Design review of the part built by this model. Coordinates are the model's own, in mm. A direction names the side the tool comes from. Round coordinates to 2 decimals unless told otherwise and drop trailing zeros. Loops run counter-clockwise (first coordinate to the right, second up) from the corner with the lowest first, then second, coordinate; pieces in that order, holes last. Notation, with made-up numbers: (0.25, 46) - (18.25, 46) arc R16 ccw to (18.25, 50) - close; hole circle Ø1 at (11.5, 62). An arc over 180 degrees is marked (long way). Use one line per item in the form item = value. Start each with the question number.
(1) For pin 1 (5 mm diameter, centred on y = -7, z = -5, fed in from -X); pin 2 (4 mm diameter, centred on x = 3, y = -5.5, fed in from -Z), all flat-tipped, find the tip position at first contact; note any pin that passes through.
(2) Wall thickness on probe 1 along Y at (x, z) = (5, 5); probe 2 along Z at (x, y) = (18.15, -5); probe 3 along Z at (x, y) = (17.75, -5.75): over which ranges is each line inside the solid? List them lowest first. Write a range as [from, to].
(3) We need section D-D, the plane z = -7.25. Write out the cut boundary in (x, y), then the cut area to 3 significant figures.
(4) The part is to be moulded in two halves that separate along Y. For faces 1 (the cylindrical face through (18.52, -5.27, -8.47)), 2 (the cylindrical face through (7.385, -4.249, 4.93)), 3 (the flat face through (10, 0, 5)), 4 (the flat face through (20, -5, 0)), say which applies: released by +Y, released by -Y, zero draft, split by the parting line, or undercut.
(5) We need section C-C, the plane x = 5. Write out the cut boundary in (y, z).
(6) Machinability: for faces 5 (the flat face through (8, -5, 0)), 6 (the flat face through (0, -5, 5)), which of the approach directions +Z, -Z, +X, -X, +Y, -Y give a long, thin tool a straight path to every point of the face, cutting with its end or side? Answer none if there is none.
(7) We need section A-A, the plane y = -5. Write out the cut boundary in (x, z), then the cut area to 4 significant figures.
(8) We need section B-B, the plane z = 7. Write out the cut boundary in (x, y), then the cut area to 3 significant figures.
from build123d import *

# Parameters (mm, degrees)
F0_W     = 20
F0_H     = 10
F0_R     = 2.5
F1_DEPTH = 10
F2_W     = 3
F2_H     = 10
F3_DEPTH = 10
F4_R     = 1.25
F5_DEPTH = 3


with BuildPart() as f1:
    # F0 (on Top) → F1 (new body)
    with BuildSketch(Plane.XY):
        with Locations((10, -5)):
            Rectangle(F0_W, F0_H)
        with Locations((5, -5)):
            Circle(F0_R, mode=Mode.SUBTRACT)
    extrude(amount=F1_DEPTH)

    # F2 (on face) → F3 (join)
    with BuildSketch(Plane(origin=(0, 0, 0), x_dir=(1, 0, 0), z_dir=(0, 0, -1))):
        with Locations((18.5, 5)):
            Rectangle(F2_W, F2_H)
    extrude(amount=F3_DEPTH)

    # F4 (on face) → F5 (cut, through all)
    with BuildSketch(Plane.YZ.offset(20)):
        with Locations((-5, -7.25)):
            Circle(F4_R)
    extrude(amount=-F5_DEPTH, mode=Mode.SUBTRACT)


solid = f1.part
Data:
q1.pin_1 = 17
q1.pin_2 = 0
q2.probe_1 = [-10, -7.5], [-2.5, 0]
q2.probe_2 = [-10, -8.5], [-6, 10]
q2.probe_3 = [-10, -8.25], [-6.25, 10]
q3.outline = (17, -10) - (20, -10) - (20, -6.25) - (17, -6.25) - close; (17, -3.75) - (20, -3.75) - (20, 0) - (17, 0) - close
q3.area = 22.5 mm^2
q4.face_1 = undercut
q4.face_2 = undercut
q4.face_3 = released by +Y
q4.face_4 = zero draft
q5.outline = (-10, 0) - (-7.5, 0) - (-7.5, 10) - (-10, 10) - close; (-2.5, 0) - (0, 0) - (0, 10) - (-2.5, 10) - close
q6.face_5 = -Z, -X, +Y, -Y
q6.face_6 = +Z, -Z, -X, +Y, -Y
q7.outline = (0, 0) - (2.5, 0) - (2.5, 10) - (0, 10) - close; (7.5, 0) - (17, 0) - (17, -6) - (20, -6) - (20, 10) - (7.5, 10) - close; (17, -10) - (20, -10) - (20, -8.5) - (17, -8.5) - close
q7.area = 172.5 mm^2
q8.outline = (0, -10) - (20, -10) - (20, 0) - (0, 0) - close; hole circle Ø5 at (5, -5)
q8.area = 180 mm^2
